For this review, use the dimensioned drawing (mm, ordinates from the lowest corner) and the shaded views. A direction names the side the tool comes from. Round coordinates to 2 decimals unless told otherwise and drop trailing zeros. Write each loop counter-clockwise with the first axis right and the second up, starting at its lowest first coordinate (ties: lowest second). Pieces come first, ordered by that corner, then holes.
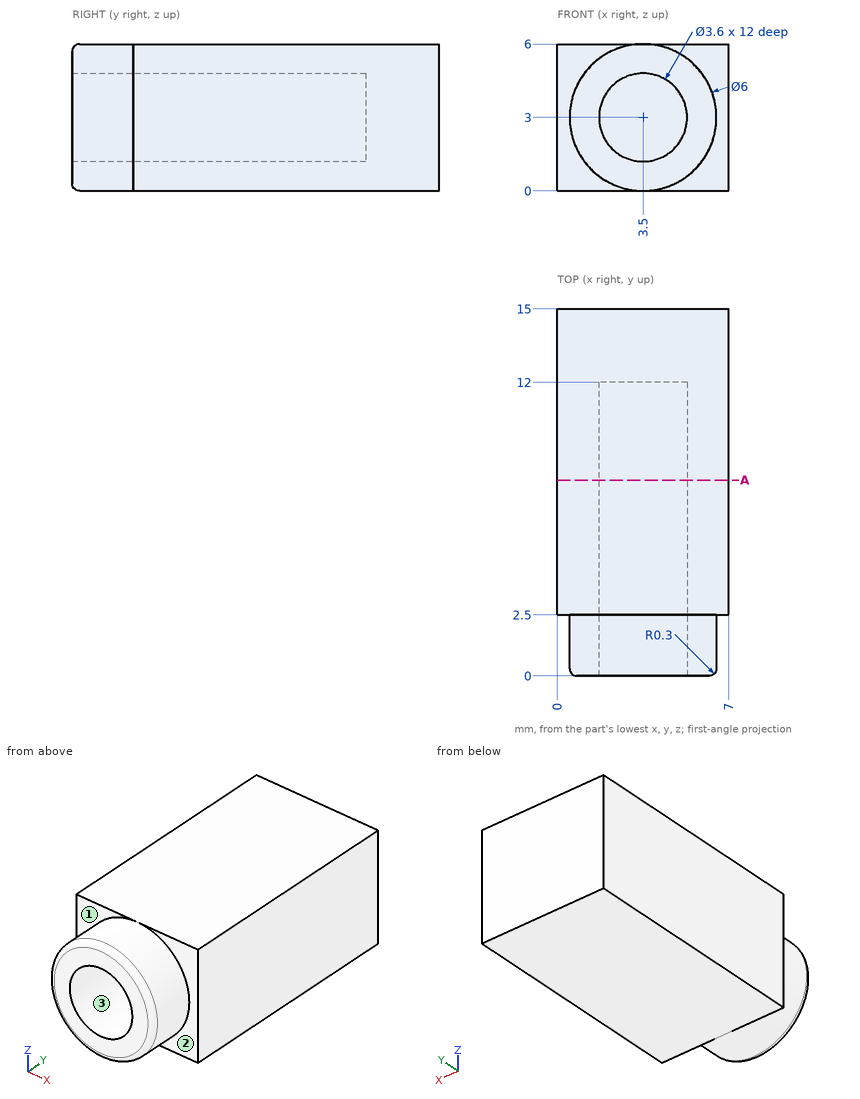
(1) We need section A-A, the plane y = 8. Give the boundary of the cut face in (x, z).
Geometry check:
outline: (0, 0) - (7, 0) - (7, 6) - (0, 6) - close; hole circle Ø3.6 at (3.5, 3)
(2) For the marked faces 1, 2 and 3, list the 3-axis set-ups (+Z, -Z, +X, -X, +Y, -Y) from which the entire face can be reached by the end or side of a thin tool; tool diameter is ignored.
Geometry check:
face 1: -X, -Y
face 2: +X, -Y
face 3: -Y
(3) For line 1 along Z through (x, y) = (3.5, 5.75); line 2 along Z through (x, y) = (3, 4.5); line 3 along X through (y, z) = (3.75, 4.25), list the stretches that pass through material, from the lowest coordinate up.
Geometry check:
line 1: z = 0 to 1.2, 4.8 to 6
line 2: z = 0 to 1.27, 4.73 to 6
line 3: x = 0 to 2.2, 4.8 to 7
(4) For pin 1 Ø1.8 at (x, z) = (4, 2.5) entering from -Y, flat-tipped, find the tip position at first contact; note if it passes through.
Geometry check:
pin 1: stops at y = 12
